For this review, take the finished solid that the model builds, in its own axes (mm). A direction names the side the tool comes from. Round coordinates to 2 decimals unless told otherwise and drop trailing zeros. Loops run counter-clockwise (first coordinate to the right, second up) from the corner with the lowest first, then second, coordinate; pieces in that order, holes last.
1) Take a section at B-B (x = 21.5). State the section outline as (y, z) points, then the cut area to 3 significant figures.
2) Take a section at C-C (z = -6). State the section outline as (x, y) points.
3) Mouldability with a two-part tool opening along X and no side actions: class faces 1 (the flat face through (25, 8.5, -3.8)), 2 (the cylindrical face through (15.504, 2.465, -13.962)), 3 (the flat face through (0, 5, -18)), 4 (the flat face through (12, 16, 12)) as pulls with the +X half, pulls with the -X half, needs draft (parallel to the pull), parting line crosses it, or undercut.
4) Tool access review of faces 5 (the flat face through (17, 16, 9.5)), 6 (the flat face through (-10, 2, 2)), 7 (the flat face through (18, -15, 4)), 8 (the flat face through (7, 7, 0)): name each direction out of +Z, -Z, +X, -X, +Y, -Y from which nothing blocks a thin tool from reaching the whole face with its end or side.
5) Wall thickness on L1, parallel to X at y = 3.1, z = -15; L2, parallel to X at y = 3, z = -22.5; L3, parallel to Z at x = 13, y = 20: over which ranges is each line inside the solid? List them lowest first.
6) Take a section at D-D (y = 43). State the section outline as (x, z) points, then the cut area to 4 significant figures.
7) Insertion check: pin 1 (6.5 mm diameter, centred on x = -12.5, z = -22.5, fed in from -Y); pin 2 (1.5 mm diameter, centred on y = 28, z = 8, fed in from -X); pin 3 (17.5 mm diameter, centred on x = 12, y = 20.5, fed in from +Z); pin 4 (2.5 mm diameter, centred on x = -10, y = 1.5, fed in from +Z). Each pin has a flat end and moves straight along its axis. Give the tip position at first contact, or say it passes through.
8) Take a section at A-A (y = 33). State the section outline as (x, z) points, then the cut area to 4 significant figures.
```python
from build123d import *

# Parameters (mm, degrees)
SKETCH1_R                = 2.8
SKETCH1_R_2              = 2.25
BOSS_EXTRUDE1_DEPTH      = 5
SKETCH3_W                = 50
SKETCH3_H                = 10
BOSS_EXTRUDE3_DEPTH      = 35
SKETCH4_R                = 2.5
CUT_EXTRUDE1_DEPTH       = 64.158530699
CHAMFER1_SIZE            = 0.75
BOSS_EXTRUDE4_DEPTH      = 30
BOSS_EXTRUDE4_DEPTH_BACK = 60
SKETCH5_W                = 10
SKETCH5_H                = 3
CHAMFER2_SIZE            = 10
CHAMFER3_SIZE            = 5
SKETCH7_W                = 2
SKETCH7_H                = 30
CUT_EXTRUDE2_DEPTH       = 88.749643874


with BuildPart() as part:
    # Sketch1 → Boss-Extrude1 (new body)
    with BuildSketch(Plane(origin=(0, 0, 0), x_dir=(1, 0, 0), z_dir=(0, 1, 0))):
        Polygon((-25, 0), (-25, 40), (25, 40), (25, 0), (25, -2), (-25, -2), align=None)
        with Locations(Location((-12.5, 22.5, 0), (0, 0, 270))):
            Circle(SKETCH1_R, mode=Mode.SUBTRACT)
        with Locations(Location((12.5, 22.5, 0), (0, 0, 270))):
            Circle(SKETCH1_R, mode=Mode.SUBTRACT)
        with Locations(Location((-17.5, 15, 0), (0, 0, 270))):
            Circle(SKETCH1_R_2, mode=Mode.SUBTRACT)
        with Locations(Location((17.5, 15, 0), (0, 0, 270))):
            Circle(SKETCH1_R_2, mode=Mode.SUBTRACT)
        with Locations(Location((0, 6, 0), (0, 0, 270))):
            Circle(SKETCH1_R, mode=Mode.SUBTRACT)
    extrude(amount=BOSS_EXTRUDE1_DEPTH)

    # Sketch3 → Boss-Extrude3 (add)
    with BuildSketch(Plane(origin=(0, 5, 0), x_dir=(1, 0, 0), z_dir=(0, 1, 0))):
        with Locations((0, 35)):
            Rectangle(SKETCH3_W, SKETCH3_H)
    extrude(amount=BOSS_EXTRUDE3_DEPTH)

    # Sketch4 → Cut-Extrude1 (cut, through all)
    with BuildSketch(Plane(origin=(0, 0, -40), x_dir=(-1, 0, 0), z_dir=(0, 0, -1))):
        with Locations((-17.8, 33)):
            Circle(SKETCH4_R)
        with Locations((17.8, 33)):
            Circle(SKETCH4_R)
    extrude(amount=-CUT_EXTRUDE1_DEPTH, mode=Mode.SUBTRACT)

    # Chamfer1
    chamfer1_edges = [part.edges().sort_by_distance(p)[0] for p in [
        (-12.5, 5, -25.3),
        (12.5, 5, -25.3),
        (0, 5, -8.8),
    ]]
    chamfer(chamfer1_edges, length=CHAMFER1_SIZE)

    # Sketch5 → Boss-Extrude4 (add, two sides: drawn at the far end of the back side and taken through both)
    with BuildSketch(Plane.XZ.offset(-BOSS_EXTRUDE4_DEPTH_BACK)):
        Polygon((13, 13), (10, 10), (10, 2), (25, 2), (25, 13), align=None)
        with Locations((17.5, 8)):
            Rectangle(SKETCH5_W, SKETCH5_H, mode=Mode.SUBTRACT)
    extrude(amount=BOSS_EXTRUDE4_DEPTH + BOSS_EXTRUDE4_DEPTH_BACK)

    # Chamfer2
    chamfer2_edges = [part.edges().sort_by_distance(p)[0] for p in [
        (17.5, 5, 2),
    ]]
    chamfer(chamfer2_edges, length=CHAMFER2_SIZE)

    # Chamfer3
    chamfer3_edges = [part.edges().sort_by_distance(p)[0] for p in [
        (10, 2.5, 2),
        (10, 5, -3),
    ]]
    chamfer(chamfer3_edges, length=CHAMFER3_SIZE)

    # Sketch7 → Cut-Extrude2 (cut, through all)
    with BuildSketch(Plane(origin=(25, 0, 0), x_dir=(0, 0, -1), z_dir=(1, 0, 0))):
        with Locations((-3, -15)):
            Rectangle(SKETCH7_W, SKETCH7_H)
    extrude(amount=-CUT_EXTRUDE2_DEPTH, mode=Mode.SUBTRACT)


solid = part.part
```
Response:
1. outline: (-30, 4) - (0, 4) - (0, -40) - (40, -40) - (40, -30) - (5, -30) - (5, -8) - (15, 2) - (60, 2) - (60, 6.5) - (-30, 6.5) - close; (-30, 9.5) - (60, 9.5) - (60, 13) - (-30, 13) - close
1. area: 1,270 mm2
2. outline: (-25, 0) - (-2.8, 0) - (-2.8, 4.25) - (-3.55, 5) - (-25, 5) - close; (2.8, 0) - (25, 0) - (25, 7) - (7, 7) - (5, 5) - (3.55, 5) - (2.8, 4.25) - close
3. face 1: pulls with the +X half
3. face 2: undercut
3. face 3: needs draft
3. face 4: pulls with the -X half
4. face 5: +Y, -Y
4. face 6: +Z, -X, +Y, -Y
4. face 7: -Z, +X, -X, -Y
4. face 8: +Z, -X, +Y
5. L1: x = -25 to -19.75, -15.25 to 15.25, 19.75 to 25
5. L2: x = -25 to -15.3, -9.7 to 9.7, 15.3 to 25
5. L3: z = -40 to -30, 2 to 6.5, 9.5 to 13
6. outline: (10, 2) - (25, 2) - (25, 13) - (13, 13) - (10, 10) - close; hole (12.5, 6.5) - (22.5, 6.5) - (22.5, 9.5) - (12.5, 9.5) - close
6. area: 130.5 mm2
7. pin 1: stops at y = 0
7. pin 2: stops at x = 10
7. pin 3: stops at z = 13
7. pin 4: stops at z = 2
8. outline: (-25, -40) - (-20.3, -40) - (-20.3, -30) - (-25, -30) - close; (-15.3, -40) - (15.3, -40) - (15.3, -30) - (-15.3, -30) - close; (10, 2) - (25, 2) - (25, 13) - (13, 13) - (10, 10) - close; (20.3, -40) - (25, -40) - (25, -30) - (20.3, -30) - close; hole (12.5, 6.5) - (22.5, 6.5) - (22.5, 9.5) - (12.5, 9.5) - close
8. area: 530.5 mm2
